```python
from build123d import *

# Parameters (mm, degrees)
PAD_DEPTH            = 20
SKETCH001_W          = 30
SKETCH001_H          = 10
PAD001_DEPTH         = 30
PAD001_DEPTH_BACK    = 20
FILLET_R             = 3
FILLET001_R          = 24
FILLET002_R          = 12
SKETCH002_R          = 3.1
POCKET_DEPTH         = 10.001
SKETCH003_R          = 5.65
POCKET001_DEPTH      = 5.6
POCKET001_DEPTH_BACK = 5
POCKET002_DEPTH      = 20.001
FILLET003_R          = 22
FILLET004_R          = 22
SKETCH005_W          = 8
SKETCH005_H          = 10.5
SKETCH005_H_2        = 30.5
PAD002_DEPTH         = 2


with BuildPart() as part:
    # Sketch → Pad (new body)
    with BuildSketch(Plane.XY):
        Polygon((-146.776695, 176.776695), (30, 0), (0, 0), (-176.776695, 176.776695), (-176.776695, 196.776695), (-146.776695, 196.776695), align=None)
        with BuildLine():
            ThreePointArc((-144.877384, 163.821067), (-148.821067, 163.821067), (-148.821067, 159.877384))
            Line((-148.821067, 159.877384), (-15.014124, 26.070441))
            ThreePointArc((-15.014124, 26.070441), (-11.070441, 26.070441), (-11.070441, 30.014124))
            Line((-144.877384, 163.821067), (-11.070441, 30.014124))
        make_face(mode=Mode.SUBTRACT)
    extrude(amount=PAD_DEPTH)

    # Sketch001 (on Face12 of Pad) → Pad001 (join, two sides)
    with BuildSketch(Plane.XY.offset(20)) as pad001_sk:
        with Locations((15, 5)):
            Rectangle(SKETCH001_W, SKETCH001_H)
    extrude(amount=PAD001_DEPTH)
    extrude(pad001_sk.sketch, amount=-PAD001_DEPTH_BACK)

    # Fillet
    fillet_edges = [part.edges().sort_by_distance(p)[0] for p in [
        (0, 5, 20),
    ]]
    fillet(fillet_edges, radius=FILLET_R)

    # Fillet001
    fillet001_edges = [part.edges().sort_by_distance(p)[0] for p in [
        (20, 10, 10),
    ]]
    fillet(fillet001_edges, radius=FILLET001_R)

    # Fillet002
    fillet002_edges = [part.edges().sort_by_distance(p)[0] for p in [
        (8.5, 10, 20),
    ]]
    fillet(fillet002_edges, radius=FILLET002_R)

    # Sketch002 (on Face1 of Fillet002) → Pocket (cut, through all)
    with BuildSketch(Plane(origin=(0, 10, 0), x_dir=(-1, 0, 0), z_dir=(0, 1, 0))):
        with Locations((-15, 35)):
            Circle(SKETCH002_R)
    extrude(amount=-POCKET_DEPTH, mode=Mode.SUBTRACT)

    # Sketch003 (on Face1 of Pocket) → Pocket001 (cut, two sides)
    with BuildSketch(Plane(origin=(0, 10, 0), x_dir=(-1, 0, 0), z_dir=(0, 1, 0))) as pocket001_sk:
        with Locations((-15, 35)):
            Circle(SKETCH003_R)
    extrude(amount=-POCKET001_DEPTH, mode=Mode.SUBTRACT)
    extrude(pocket001_sk.sketch, amount=POCKET001_DEPTH_BACK, mode=Mode.SUBTRACT)

    # Sketch004 (on Face21 of Pocket001) → Pocket002 (cut, through all)
    with BuildSketch(Plane.XY.offset(20)):
        with BuildLine():
            ThreePointArc((-157.626695, 204.776695), (-161.776695, 208.926695), (-165.926695, 204.776695))
            Line((-165.926695, 204.776695), (-165.926695, 188.776695))
            ThreePointArc((-165.926695, 188.776695), (-161.776695, 184.626695), (-157.626695, 188.776695))
            Line((-157.626695, 204.776695), (-157.626695, 188.776695))
        make_face()
    extrude(amount=-POCKET002_DEPTH, mode=Mode.SUBTRACT)

    # Fillet003
    fillet003_edges = [part.edges().sort_by_distance(p)[0] for p in [
        (-146.776695, 176.776695, 10),
    ]]
    fillet(fillet003_edges, radius=FILLET003_R)

    # Fillet004
    fillet004_edges = [part.edges().sort_by_distance(p)[0] for p in [
        (-176.776695, 176.776695, 10),
    ]]
    fillet(fillet004_edges, radius=FILLET004_R)

    # Sketch005 (on Face4 of Fillet004) → Pad002 (join)
    with BuildSketch(Plane.XZ):
        with Locations((15, 44.75)):
            Rectangle(SKETCH005_W, SKETCH005_H)
        with Locations((15, 15.25)):
            Rectangle(SKETCH005_W, SKETCH005_H_2)
    extrude(amount=PAD002_DEPTH)


solid = part.part
```
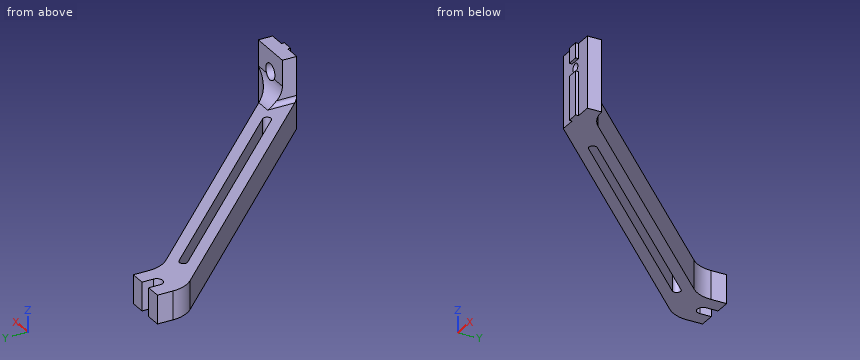
Model file for the job. Use its own axes, mm. Coordinates: 2 decimals unless noted, no trailing zeros. Write each loop counter-clockwise with the first axis right and the second up, starting at its lowest first coordinate (ties: lowest second). Pieces come first, ordered by that corner, then holes. Notation, with made-up numbers: (39, 32.25) - (55, 32.25) arc R26 ccw to (55, 63.25) - close; hole circle Ø3 at (79.5, -23). An arc over 180 degrees is marked (long way). Use a Markdown table: item, result. Add a question column.
Item 1: Drop flat-ended pins along their axis: pin 1 (8 mm diameter, centred on x = -55.5, y = 90.5, fed in from +Z); pin 2 (24 mm diameter, centred on x = 20, z = 37.5, fed in from +Y); pin 3 (7 mm diameter, centred on y = 6.5, z = 32.5, fed in from -X); pin 4 (12 mm diameter, centred on x = -152, y = 135.5, fed in from +Z). Give the stop position or say it passes through.
Item 2: Band-saw the part on C-C, the plane z = 7. Write the cut outline in (x, y).
Item 3: Band-saw the part on A-A, the plane z = 35. Write the cut outline in (x, y), and give its area (3 significant figures).
Item 4: Band-saw the part on B-B, the plane x = -63.5. Write the cut outline in (y, z), and give its area (3 significant figures).
Item 5: Band-saw the part on D-D, the plane y = 103. Write the cut outline in (x, z), and give its area (3 significant figures).
Item 6: Drill centre lines: line 1 along Z through (x, y) = (15, 2.2); line 2 along X through (y, z) = (6, 35); line 3 along Y through (x, z) = (-69.5, 5). Where is each one in solid material? Low to high.
A:
| question | item | result |
|---|---|---|
| 1 | pin 1 | stops at z = 20 |
| 1 | pin 2 | stops at y = 11.91 |
| 1 | pin 3 | stops at x = 0 |
| 1 | pin 4 | passes through |
| 2 | outline | (-176.78, 185.89) arc R22 ccw to (-170.33, 170.33) - (0, 0) - (11, 0) - (11, -2) - (19, -2) - (19, 0) - (30, 0) - (30, 10) - (29.94, 10) arc R24 cw to (12.97, 17.03) - (-140.33, 170.33) arc R22 cw to (-146.78, 185.89) - (-146.78, 196.78) - (-157.63, 196.78) - (-157.63, 188.78) arc R4.15 cw to (-165.93, 188.78) - (-165.93, 196.78) - (-176.78, 196.78) - close; hole (-148.82, 159.88) - (-15.01, 26.07) arc R2.79 ccw to (-11.07, 30.01) - (-144.88, 163.82) arc R2.79 ccw to start |
| 3 | outline | (0, 0) - (11.9, 0) - (11.9, 4.4) - (9.35, 4.4) - (9.35, 10) - (0, 10) - close; (18.1, 0) - (30, 0) - (30, 10) - (20.65, 10) - (20.65, 4.4) - (18.1, 4.4) - close |
| 3 | area | 209 mm² |
| 4 | outline | (63.5, 0) - (74.56, 0) - (74.56, 20) - (63.5, 20) - close; (82.44, 0) - (93.5, 0) - (93.5, 20) - (82.44, 20) - close |
| 4 | area | 442 mm² |
| 5 | outline | (-103, 0) - (-91.94, 0) - (-91.94, 20) - (-103, 20) - close; (-84.06, 0) - (-73, 0) - (-73, 20) - (-84.06, 20) - close |
| 5 | area | 442 mm² |
| 6 | line 1 | z = 0 to 31.9, 38.1 to 50 |
| 6 | line 2 | x = 0 to 9.35, 20.65 to 30 |
| 6 | line 3 | y = 69.5 to 80.56, 88.44 to 99.5 |
